from build123d import *

# Parameters (mm, degrees)
F0_W     = 12.690173
F0_H     = 11.43
F1_DEPTH = 101.6
F3_DEPTH = 25.4
F6_D     = 7.62
F6_DEPTH = 19.05
F7_D     = 7.62
F7_DEPTH = 19.05


with BuildPart() as f1:
    # F0 (on Front) → F1 (new body)
    with BuildSketch(Plane.XZ):
        with Locations((-6.345086, 5.715)):
            Rectangle(F0_W, F0_H)
    extrude(amount=F1_DEPTH)

    # F2 (on face) → F3 (cut)
    with BuildSketch(Plane(origin=(-12.690173, 0, 0), x_dir=(0, -1, 0), z_dir=(-1, 0, 0))):
        Polygon((50.8, 11.43), (48.294391, 11.43), (50.8, 6.035571), (56.032304, 6.035571), (56.032304, 11.43), align=None)
    extrude(amount=-F3_DEPTH, mode=Mode.SUBTRACT)

    # F6
    with Locations(Plane(origin=(-12.690173, 0, 0), x_dir=(0, -1, 0), z_dir=(-1, 0, 0))):
        with Locations((8.057253, 5.715)):
            Hole(F6_D / 2, depth=F6_DEPTH)

    # F7
    with Locations(Plane(origin=(-12.690173, 0, 0), x_dir=(0, -1, 0), z_dir=(-1, 0, 0))):
        with Locations((93.793303, 5.726054)):
            Hole(F7_D / 2, depth=F7_DEPTH)


solid = f1.part
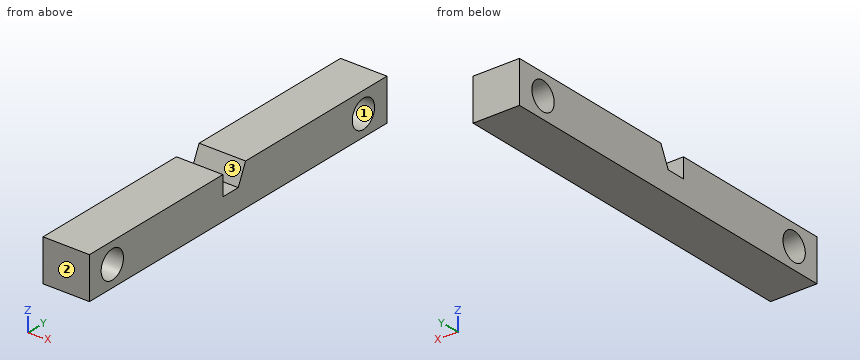
Can you work these out from the model? Positions are in its coordinate system, mm. Face numbers are marked on the shaded views. Coordinates: 2 decimals unless noted, no trailing zeros. Order: outer loops, then holes, each group sorted by start corner. A loop starts at its lowest first (then second) coordinate and runs counter-clockwise, first axis right, second up. Notation, with made-up numbers: M 32,75.5 L 43,75.5 A32 ccw 43,101.5 Z; hole C -24.75,76 d2. An arc over 180 degrees is marked long. Write item = value, one per line.
(1) Suppose I cut it at D-D on y = -10. Please give me the cut outline in (x, z), plus the area to 3 significant figures.
Results are:
outline = M -12.69,0 L 0,0 L 0,2.44 L -12.69,2.44 Z; M -12.69,8.99 L 0,8.99 L 0,11.43 L -12.69,11.43 Z
area = 61.9 mm2
(2) Suppose I cut it at B-B on y = -91. Please give me the cut outline in (x, z) (3 decimals), plus the area to 3 significant figures.
Results are:
outline = M -12.69,0 L 0,0 L 0,3.135 L -12.69,3.135 Z; M -12.69,8.317 L 0,8.317 L 0,11.43 L -12.69,11.43 Z
area = 79.3 mm2
(3) Suppose I cut it at C-C on x = -3.75. Please give me the cut outline in (y, z) (3 decimals).
Results are:
outline = M -101.6,0 L 0,0 L 0,11.43 L -48.294,11.43 L -50.8,6.036 L -56.032,6.036 L -56.032,11.43 L -101.6,11.43 Z; hole C -93.793,5.726 d7.62; hole C -8.057,5.715 d7.62
(4) I need wall thicknesses on line 1 along Y through (x, z) = (-2.5, 6); line 2 along Y through (x, z) = (-10.5, 7.5); line 3 along Y through (x, z) = (-4.25, 4.75). Which ranges of each line are inside material? Lowest first, please. Write a range as [from, to].
Results are:
line_1 = [-101.6, -97.59], [-89.99, -11.86], [-4.26, 0]
line_2 = [-101.6, -97.17], [-90.42, -56.03], [-50.12, -11.42], [-4.69, 0]
line_3 = [-101.6, -97.48], [-90.11, -11.74], [-4.37, 0]
(5) For pin 1 Ø4.5 at (x, z) = (-3.5, 8.5) entering from +Y; pin 2 Ø4 at (x, y) = (-7.5, -52.5) entering from +Z, each with a flat end and sliding along its axis, tell me the tip position at first contact or that it passes through.
Results are:
pin_1 = 0
pin_2 = 6.68
(6) Suppose I cut it at A-A on z = 4.75. Please give me the cut outline in (x, y).
Results are:
outline = M -12.69,-101.6 L 0,-101.6 L 0,-97.48 L -12.69,-97.48 Z; M -12.69,-90.11 L 0,-90.11 L 0,-11.74 L -12.69,-11.74 Z; M -12.69,-4.37 L 0,-4.37 L 0,0 L -12.69,0 Z
(7) If we mould it in two halves opening along Z, with no side actions, what happens to the marked faces 1, 2 and 3? For each: pulls with the +Z half, pulls with the -Z half, needs draft (parallel to the pull), parting line crosses it, or undercut.
Results are:
face_1 = undercut
face_2 = needs draft
face_3 = pulls with the +Z half
